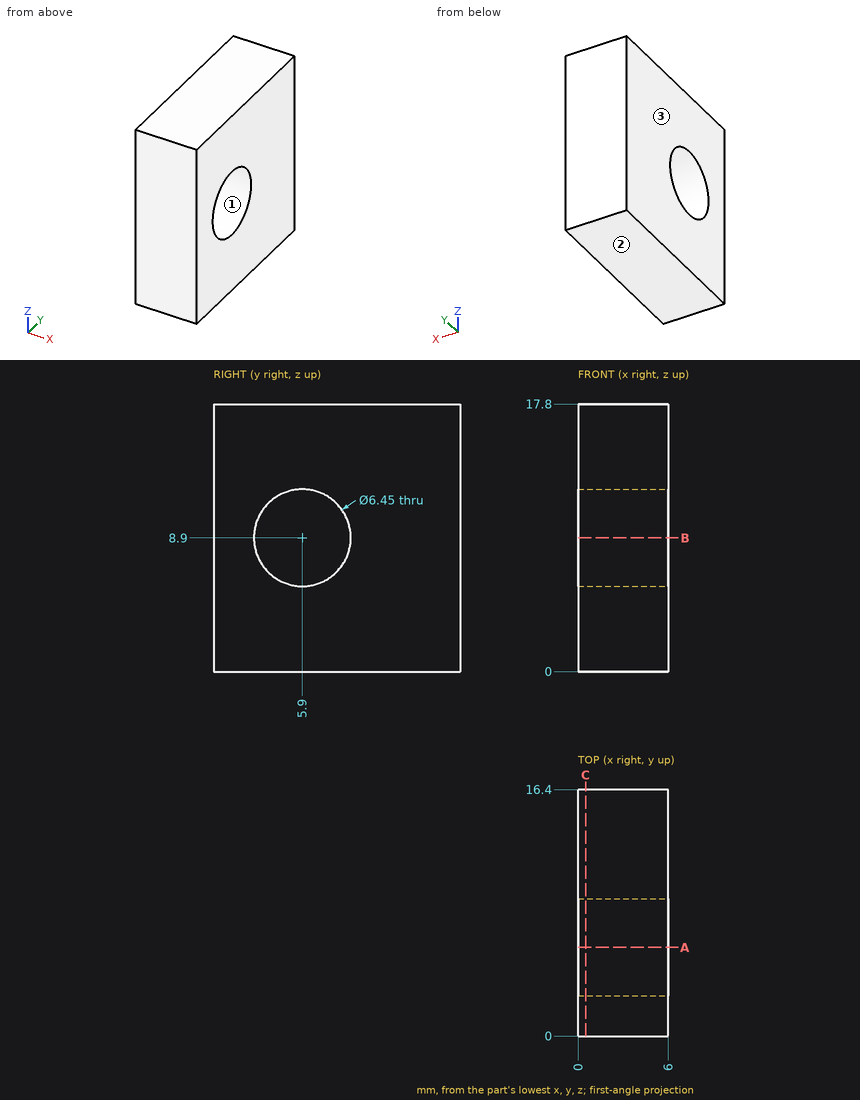
Here's the drawing with two shaded views (mm, measured from the low corner). I have some questions. Give positions to 0.01 mm unless a question says otherwise; leave off trailing zeros. Write each loop counter-clockwise with the first axis right and the second up, starting at its lowest first coordinate (ties: lowest second). Pieces come first, ordered by that corner, then holes. Notation, with made-up numbers: (-22, -37) - (25, -37) arc R20 cw to (25, -28) - close; hole circle Ø5 at (-29, 30). An arc over 180 degrees is marked (long way). Write item = value, one per line. Start each with the question number.
1. Thinking about a two-plate mould opening in Z: for the marked faces 1, 2 and 3, which applies, released by +Z, released by -Z, zero draft, split by the parting line, or undercut?
2. Imagine slicing it at C-C (x = 0.5). Please give me the cut outline in (y, z) (3 decimals), and give its area (3 significant figures).
3. Imagine slicing it at B-B (z = 8.9). Please give me the cut outline in (x, y) (3 decimals).
4. Imagine slicing it at A-A (y = 5.9). Please give me the cut outline in (x, z) (3 decimals), and give its area (3 significant figures).
5. Please list where these lines run through material, in increasing order: line 1 (Y direction, x = 3.8, z = 8.9) (3 decimals); line 2 (Z direction, x = 2.8, y = 7); line 3 (Y direction, x = 3.4, z = 6).
6. For pin 1 (8 mm diameter, centred on y = 10.5, z = 11.5, fed in from -X), with a flat end and sliding along its axis, tell me the tip position at first contact or that it passes through.
Worked answers:
q1.face_1 = undercut
q1.face_2 = released by -Z
q1.face_3 = zero draft
q2.outline = (0, 0) - (16.4, 0) - (16.4, 17.8) - (0, 17.8) - close; hole circle Ø6.45 at (5.9, 8.9)
q2.area = 259 mm2
q3.outline = (0, 0) - (6, 0) - (6, 2.675) - (0, 2.675) - close; (0, 9.125) - (6, 9.125) - (6, 16.4) - (0, 16.4) - close
q4.outline = (0, 0) - (6, 0) - (6, 5.675) - (0, 5.675) - close; (0, 12.125) - (6, 12.125) - (6, 17.8) - (0, 17.8) - close
q4.area = 68.1 mm2
q5.line_1 = 0 to 2.675, 9.125 to 16.4
q5.line_2 = 0 to 5.87, 11.93 to 17.8
q5.line_3 = 0 to 4.49, 7.31 to 16.4
q6.pin_1 = 0
